```python
from build123d import *

# Parameters (mm, degrees)
F1_DEPTH = 6.35


with BuildPart() as f1:
    # F0 (on Front) → F1 (new body)
    with BuildSketch(Plane.XZ):
        with BuildLine():
            Line((155.086583, 34.469813), (-79.863417, 34.469813))
            Line((-79.863417, 34.469813), (-79.863417, 15.419813))
            Line((-79.863417, 15.419813), (-75.100917, 15.419813))
            ThreePointArc((-75.100917, 15.419813), (-73.513417, 17.007313), (-71.925917, 15.419813))
            ThreePointArc((-71.925917, 15.419813), (-72.390885, 14.297281), (-73.513417, 13.832313))
            Line((-73.513417, 13.832313), (-73.513417, -2.042687))
            ThreePointArc((-73.513417, -2.042687), (-72.390885, -2.507655), (-71.925917, -3.630187))
            ThreePointArc((-71.925917, -3.630187), (-73.513417, -5.217687), (-75.100917, -3.630187))
            Line((-75.100917, -3.630187), (-79.863417, -3.630187))
            Line((-79.863417, -3.630187), (-79.863417, -16.330187))
            Line((-79.863417, -16.330187), (-49.700917, -16.330187))
            ThreePointArc((-49.700917, -16.330187), (-48.113417, -14.742687), (-46.525917, -16.330187))
            Line((-46.525917, -16.330187), (-30.650917, -16.330187))
            ThreePointArc((-30.650917, -16.330187), (-29.063417, -14.742687), (-27.475917, -16.330187))
            Line((-27.475917, -16.330187), (26.499083, -16.330187))
            ThreePointArc((26.499083, -16.330187), (28.086583, -14.742687), (29.674083, -16.330187))
            Line((29.674083, -16.330187), (45.549083, -16.330187))
            ThreePointArc((45.549083, -16.330187), (47.136583, -14.742687), (48.724083, -16.330187))
            Line((48.724083, -16.330187), (102.699083, -16.330187))
            ThreePointArc((102.699083, -16.330187), (104.286583, -14.742687), (105.874083, -16.330187))
            Line((105.874083, -16.330187), (121.749083, -16.330187))
            ThreePointArc((121.749083, -16.330187), (123.336583, -14.742687), (124.924083, -16.330187))
            Line((124.924083, -16.330187), (155.086583, -16.330187))
            Line((155.086583, -16.330187), (155.086583, -3.630187))
            Line((155.086583, -3.630187), (150.324083, -3.630187))
            ThreePointArc((150.324083, -3.630187), (147.614051, -4.752719), (148.736583, -2.042687))
            Line((148.736583, -2.042687), (148.736583, 13.832313))
            ThreePointArc((148.736583, 13.832313), (147.614051, 16.542345), (150.324083, 15.419813))
            Line((150.324083, 15.419813), (155.086583, 15.419813))
            Line((155.086583, 15.419813), (155.086583, 34.469813))
        make_face()
        with BuildLine():
            ThreePointArc((-3.663417, 13.832313), (-4.785949, 16.542345), (-2.075917, 15.419813))
            Line((-2.075917, 15.419813), (1.099083, 15.419813))
            ThreePointArc((1.099083, 15.419813), (2.686583, 17.007313), (4.274083, 15.419813))
            ThreePointArc((4.274083, 15.419813), (3.809115, 14.297281), (2.686583, 13.832313))
            Line((2.686583, 13.832313), (2.686583, -2.042687))
            ThreePointArc((2.686583, -2.042687), (3.809115, -2.507655), (4.274083, -3.630187))
            ThreePointArc((4.274083, -3.630187), (2.686583, -5.217687), (1.099083, -3.630187))
            Line((1.099083, -3.630187), (-2.075917, -3.630187))
            ThreePointArc((-2.075917, -3.630187), (-4.785949, -4.752719), (-3.663417, -2.042687))
            Line((-3.663417, -2.042687), (-3.663417, 13.832313))
        make_face(mode=Mode.SUBTRACT)
        with BuildLine():
            ThreePointArc((72.536583, 13.832313), (71.414051, 16.542345), (74.124083, 15.419813))
            Line((74.124083, 15.419813), (77.299083, 15.419813))
            ThreePointArc((77.299083, 15.419813), (78.886583, 17.007313), (80.474083, 15.419813))
            ThreePointArc((80.474083, 15.419813), (80.009115, 14.297281), (78.886583, 13.832313))
            Line((78.886583, 13.832313), (78.886583, -2.042687))
            ThreePointArc((78.886583, -2.042687), (80.009115, -2.507655), (80.474083, -3.630187))
            ThreePointArc((80.474083, -3.630187), (78.886583, -5.217687), (77.299083, -3.630187))
            Line((77.299083, -3.630187), (74.124083, -3.630187))
            ThreePointArc((74.124083, -3.630187), (71.414051, -4.752719), (72.536583, -2.042687))
            Line((72.536583, -2.042687), (72.536583, 13.832313))
        make_face(mode=Mode.SUBTRACT)
        with BuildLine():
            Line((-30.650917, -16.330187), (-46.525917, -16.330187))
            ThreePointArc((-46.525917, -16.330187), (-46.990885, -17.452719), (-48.113417, -17.917687))
            Line((-48.113417, -17.917687), (-48.113417, -22.680187))
            Line((-48.113417, -22.680187), (-29.063417, -22.680187))
            Line((-29.063417, -22.680187), (-29.063417, -17.917687))
            ThreePointArc((-29.063417, -17.917687), (-30.185949, -17.452719), (-30.650917, -16.330187))
        make_face()
        with BuildLine():
            Line((45.549083, -16.330187), (29.674083, -16.330187))
            ThreePointArc((29.674083, -16.330187), (29.209115, -17.452719), (28.086583, -17.917687))
            Line((28.086583, -17.917687), (28.086583, -22.680187))
            Line((28.086583, -22.680187), (47.136583, -22.680187))
            Line((47.136583, -22.680187), (47.136583, -17.917687))
            ThreePointArc((47.136583, -17.917687), (46.014051, -17.452719), (45.549083, -16.330187))
        make_face()
        with BuildLine():
            ThreePointArc((123.336583, -17.917687), (122.214051, -17.452719), (121.749083, -16.330187))
            Line((121.749083, -16.330187), (105.874083, -16.330187))
            ThreePointArc((105.874083, -16.330187), (105.409115, -17.452719), (104.286583, -17.917687))
            Line((104.286583, -17.917687), (104.286583, -22.680187))
            Line((104.286583, -22.680187), (123.336583, -22.680187))
            Line((123.336583, -22.680187), (123.336583, -17.917687))
        make_face()
    extrude(amount=F1_DEPTH)


solid = f1.part
```
Could you check a few things on this model? Use its own coordinates, in mm. A direction names the side the tool comes from. Coordinates: 2 decimals unless noted, no trailing zeros. Loops run counter-clockwise (first coordinate to the right, second up) from the corner with the lowest first, then second, coordinate; pieces in that order, holes last.
1) Imagine slicing it at B-B (y = -3.75). State how many separate pieces and enclosed holes the cut face has, and give its area (3 significant figures).
Reported:
separate pieces: 1
enclosed holes: 2
area: 11,700 mm2
2) Please list where these lines run through material, in increasing order: line 1 along X through (y, z) = (-4.5, 8.5); line 2 along Z through (x, y) = (123, -0.75); line 3 along Z through (x, y) = (6.5, -3).
Reported:
line 1: x = -73.51 to -3.66, 2.69 to 72.54, 78.89 to 148.74
line 2: z = -22.68 to -17.88, -14.78 to 34.47
line 3: z = -16.33 to 34.47
3) Imagine slicing it at C-C (x = 6.5). List the corners of the cut face in (y, z) for me, and give its area (3 significant figures).
Reported:
outline: (-6.35, -16.33) - (0, -16.33) - (0, 34.47) - (-6.35, 34.47) - close
area: 323 mm2
4) Which directions (+Z, -Z, +X, -X, +Y, -Y) give clear straight access to the entire face, cutting with the end or side of a thin tool? Please do faces 1 (the face through (-48.113, -3, -20)), 2 (the face through (-78, -3, 15.42)), 3 (the face through (140, -3, -16.33)), 4 (the face through (-3.663, -3, 6)), 5 (the face through (153, -3, -3.63)).
Reported:
face 1: -Z, -X, +Y, -Y
face 2: -X, +Y, -Y
face 3: -Z, +X, +Y, -Y
face 4: +Y, -Y
face 5: +X, +Y, -Y
5) Thinking about a two-plate mould opening in Z: for faces 6 (the face through (2.687, -3, 6)), 7 (the face through (36, 0, 6)), 8 (the face through (-1, -3, -16.33)), which applies, released by +Z, released by -Z, zero draft, split by the parting line, or undercut?
Reported:
face 6: undercut
face 7: zero draft
face 8: released by -Z
6) Will these pins go through, and if not, where does the flat tip stop? pin 1 Ø1.9 at (x, z) = (-3.66, -3.63) entering from +Y; pin 2 Ø1.9 at (y, z) = (-4, 4) entering from +X; pin 3 Ø2.5 at (y, z) = (-4, -21) entering from -X; pin 4 Ø1.4 at (y, z) = (-3, -20) entering from +X.
Reported:
pin 1: passes through
pin 2: stops at x = 148.74
pin 3: stops at x = -48.11
pin 4: stops at x = 123.34
7) Imagine slicing it at A-A (z = 4.5). List the corners of the cut face in (x, y) for me, and give its area (3 significant figures).
Reported:
outline: (-73.51, -6.35) - (-3.66, -6.35) - (-3.66, 0) - (-73.51, 0) - close; (2.69, -6.35) - (72.54, -6.35) - (72.54, 0) - (2.69, 0) - close; (78.89, -6.35) - (148.74, -6.35) - (148.74, 0) - (78.89, 0) - close
area: 1,330 mm2
